Part model, mm, in its own coordinate system. A direction names the side the tool comes from. Round coordinates to 2 decimals unless told otherwise and drop trailing zeros. Loops run counter-clockwise (first coordinate to the right, second up) from the corner with the lowest first, then second, coordinate; pieces in that order, holes last. Notation, with made-up numbers: M 77,36 L 83,36 A28 cw 83,73 Z; hole C 35.5,32.25 d4. An arc over 180 degrees is marked long. Write each question's results on one line, items separated by ' | '.
from build123d import *

# Parameters (mm, degrees)
F0_R     = 2.75
F1_DEPTH = 2


with BuildPart() as f1:
    # F0 (on Top) → F1 (new body)
    with BuildSketch(Plane.XY):
        Polygon((42.614597, 43.575729), (40.474674, 43.801061), (40.474674, 44.904759), (41.289306, 45.377769), (42.235331, 46.061014), (42.997407, 46.954477), (43.680649, 48.268405), (44.023932, 49.729318), (44.023932, 50.649449), (44.023932, 51.944449), (43.5775, 53.083367), (42.691444, 54.156854), (41.847845, 54.906591), (40.794143, 55.656328), (39.760655, 55.963038), (38.738284, 56.099354), (37.5796, 56.099354), (36.625389, 55.877841), (36.011968, 55.622249), (35.398544, 55.400736), (35.096974, 55.400736), (34.725139, 56.293141), (34.122785, 57.161563), (33.357102, 57.842052), (32.042509, 58.77742), (31.030484, 59.166825), (29.802747, 59.330523), (28.542718, 59.330523), (27.281797, 59.132746), (26.350169, 58.744568), (25.505657, 58.392688), (24.732415, 57.754455), (24.507659, 57.438576), (23.805742, 57.438576), (23.38257, 58.454189), (22.428905, 59.132746), (21.566604, 59.746296), (20.461918, 60.19183), (19.297132, 60.347135), (18.092803, 60.507712), (16.778593, 60.307712), (15.680915, 59.992126), (14.727073, 59.330523), (13.943266, 58.78686), (13.211777, 58.18309), (12.717188, 57.316541), (12.371887, 56.831245), (12.102754, 56.452998), (11.70455, 56.452998), (11.181221, 56.82536), (9.885113, 56.998174), (8.770078, 56.998174), (7.202732, 56.627827), (6.197297, 56.099354), (5.286899, 55.467885), (4.67496, 54.779335), (4.109085, 53.843544), (3.745405, 52.941812), (3.43555, 51.734029), (3.43555, 50.828029), (3.43555, 49.455927), (3.745405, 48.712276), (4.102451, 47.855367), (4.868277, 46.927541), (5.71123, 45.906275), (6.588969, 45.375504), (6.958782, 45.046838), (6.732116, 43.34684), (4.67496, 7.491453), (4.382145, 7.007223), (3.745405, 6.741914), (3.021601, 6.440329), (2.510416, 6.018397), (2.181404, 5.474309), (2.084989, 4.751196), (2.186613, 4.115137), (2.862741, 3.634054), (3.745405, 3.100305), (4.911553, 2.629983), (6.412406, 2.274872), (7.980039, 1.934082), (9.45109, 1.737943), (10.984644, 1.53347), (12.690081, 1.306079), (14.643297, 1.04565), (16.432547, 1.003336), (18.755258, 0.929009), (20.764264, 0.881497), (24.674177, 0.881497), (29.284421, 1.04565), (32.075043, 1.127764), (33.867482, 1.224696), (35.480599, 1.434622), (37.137908, 1.644548), (38.817317, 1.964962), (39.922824, 2.181308), (41.015109, 2.450639), (41.856079, 2.658001), (42.635252, 2.945225), (43.519151, 3.276687), (44.177526, 3.632565), (44.729134, 3.952855), (45.129498, 4.308733), (45.343027, 4.646817), (45.323095, 5.206614), (45.049425, 5.767831), (44.637698, 6.263237), (43.964259, 6.642941), (43.391121, 6.814882), (42.72485, 7.02981), (42.517087, 7.130109), (42.161251, 17.123776), (43.045596, 17.341834), (44.277249, 17.645529), (45.452933, 17.935424), (46.488645, 18.385407), (47.477306, 18.81526), (48.072154, 19.273718), (48.74559, 19.818199), (49.340221, 20.31253), (49.963509, 20.892833), (50.379035, 21.322686), (50.726546, 22.042045), (51.13535, 23.003285), (51.511009, 23.798795), (51.864567, 24.671646), (52.240226, 25.77652), (52.483299, 26.682517), (52.659055, 28.000691), (52.860135, 29.508797), (52.695712, 34.126613), (52.405689, 35.302818), (52.055256, 37.139574), (51.341367, 38.460271), (50.695767, 40.152436), (49.438013, 41.668941), (47.999089, 42.388402), (46.350579, 42.830686), (44.521046, 43.321537), align=None)
        Polygon((41.847845, 22.476589), (40.794143, 38.363158), (42.253113, 38.322631), (43.874192, 37.957887), (45.495268, 37.309456), (46.548973, 36.093648), (47.116347, 34.756259), (47.764781, 33.175707), (47.764781, 31.39252), (47.764781, 28.434052), (47.278455, 26.448232), (46.548973, 25.070315), (45.495268, 23.935562), (44.117352, 23.043968), (42.619834, 22.527792), align=None, mode=Mode.SUBTRACT)
        with Locations((36.087643, 40.83737)):
            Circle(F0_R, mode=Mode.SUBTRACT)
    extrude(amount=F1_DEPTH)


solid = f1.part
Item 1: Wall check: L1, parallel to X at y = 41.5, z = 1.3; L2, parallel to X at y = 29, z = 0.6; L3, parallel to Y at x = 37, z = 0.95. Give the ranges that are in metal, low to high.
Filled sheet:
L1: 6.63 to 33.42, 38.76 to 49.58 | L2: 5.91 to 41.42, 47.76 to 52.79 | L3: 1.63 to 38.24, 43.43 to 55.96
Item 2: Drop flat-ended pins along their axis: P1, Ø0.9, axis at x = 9.5, z = 1, coming from the +Y side; P2, Ø1, axis at y = 51, z = 1, coming from the -X side; P3, Ø0.6, axis at x = 29, z = 1, coming from the +Y side. Give the stop position or say it passes through.
Filled sheet:
P1: y = 57 | P2: x = 3.44 | P3: y = 59.33
Item 3: Band-saw the part on B-B on z = 0.55. Count the separate pieces of the cut face and the enclosed holes in it, and give its area (3 significant figures).
Filled sheet:
separate pieces: 1 | enclosed holes: 2 | area: 2,230 mm^2
Item 4: Band-saw the part on A-A on y = 14. Give the cut face in (x, z), and give its area (3 significant figures).
Filled sheet:
outline: M 5.05,0 L 42.27,0 L 42.27,2 L 5.05,2 Z | area: 74.4 mm^2
Item 5: Which spindle directions (+Z, -Z, +X, -X, +Y, -Y) get a long thin tool onto all of the face, cutting with end or side? Do faces 1 (the flat face through (44.67, 37.64, 0.99)), 2 (the flat face through (5.718, 25.67, 0.986)), 3 (the flat face through (29, 59.331, 1)). Say none if no direction does.
Filled sheet:
face 1: +Z, -Z | face 2: +Z, -Z, -X | face 3: +Z, -Z, +X, +Y
Item 6: Two-plate mould, pull along Y, no slides. Class faces 4 (the flat face through (43.38, 22.79, 0.99)), 5 (the flat face through (34.663, 1.328, 0.986)), 6 (the flat face through (43.581, 43.447, 0.986)), 7 (the flat face through (10.54, 56.91, 0.99)): +Y half, -Y half, draft (parallel to the pull), parting line (faces both ways), or undercut.
Filled sheet:
face 4: undercut | face 5: -Y half | face 6: undercut | face 7: +Y half
